Autodesk Inventor part; units mm, degrees
ref_plane "YZ Plane" through (0, 0, 0) normal (1, 0, 0) x (0, 1, 0)
ref_plane "XZ Plane" through (0, 0, 0) normal (0, 1, 0) x (-1, 0, 0)
ref_plane "XY Plane" through (0, 0, 0) normal (0, 0, 1) x (1, 0, 0)
sketch "Main Sketch" plane through (0, 0, 0) normal (0, 1, 0) x (-1, 0, 0)
  line L0 (-57.375, -12.0472) -> (-57.375, 12.0472)
  line L1 (-57.375, 12.0472) -> (47.625, -10) construction
  line L2 (47.625, 10) -> (-57.375, -12.0472) construction
  circle A0 centre (47.625, 0) radius 7
  line L3 (-40.875, 17.5) -> (-57.375, 17.5)
  line L4 (-57.375, 17.5) -> (-57.375, -17.5)
  line L5 (-57.375, -17.5) -> (-40.875, -17.5)
  line L6 (-40.875, 17.5) -> (-57.375, -17.5) construction
  line L7 (-57.375, 17.5) -> (-40.875, -17.5) construction
  line L8 (33.2636, -10) -> (-40.875, -10)
  line L9 (-40.875, -17.5) -> (-40.875, -10)
  line L10 (-40.875, 10) -> (-40.875, 17.5)
  line L11 (-40.875, 10) -> (33.2636, 10)
  arc A1 (33.2636, -10) -> (33.2636, 10) centre (47.625, 0) ccw
  point P0 (0, 0)
  point P1 (-49.125, 0)
  dimension "d3" = 14
  dimension "d13" = 16.5
  dimension "d14" = 35
  dimension "d15" = 0
  dimension "d18" = 20
  dimension "d101" = 35
extrude "Main Extrusion" add sketch "Main Sketch" along normal blind 4
sketch "Screw Holes Sketch" plane through (0, 4, 0) normal (0, 1, 0) x (1, 0, 0)
  circle A0 centre (46.125, -8.75) radius 2
  line L0 (57.375, 17.5) -> (40.875, 17.5)
  line L1 (40.875, -17.5) -> (57.375, -17.5)
  line L2 (35.2664, 0) -> (65.7891, 0)
  line L3 (51.375, -27.0398) -> (51.375, 30.2346) construction
  line L4 (57.375, -17.5) -> (57.375, 17.5)
  line L5 (40.875, -10) -> (40.875, -17.5)
  circle A1 centre (46.125, 8.75) radius 2
  line L6 (51.375, 27.0398) -> (51.375, -30.2346) construction
  point P0 (0, 0)
  dimension "d21" = 4
  dimension "d22" = 35
  dimension "d23" = 6
  dimension "d24" = 5.25
  dimension "d25" = 5.25
  dimension "d26" = 10.5
  dimension "d27" = 8.75
  dimension "d28" = 17.5
extrude "Screw Holes Cut" cut sketch "Screw Holes Sketch" against normal through all
fillet "Smoooooooooooooooooth" radius 6 2 edges at (40.875, 2, -17.5) (40.875, 2, 17.5)
sketch "Side Axel Hole Sketch" plane through (-47.625, 0, 10) normal (0, 0, 1) x (1, 0, 0)
  line L0 (88.5, 4) -> (88.5, 0)
  line L1 (0, 0) -> (0, 4)
  line L2 (44.25, -12.0383) -> (44.25, 22.7681) construction
  line L3 (14.3614, 0) -> (88.5, 0)
  line L4 (14.3614, 4) -> (88.5, 4)
  circle A0 centre (44.25, 4) radius 1.5
  point P0 (47.625, 0)
  dimension "d32" = 88.5
  dimension "d33" = 44.25
  dimension "d34" = 44.25
  dimension "d35" = 4
  dimension "d41" = 3
extrude "Side Axel Hole Cut" cut sketch "Side Axel Hole Sketch" against normal blind 20
sketch "Side Hole Extension Sketch" plane through (-47.625, 0, 10) normal (0, 0, 1) x (1, 0, 0)
  arc A0 (42.75, 4) -> (45.75, 4) centre (44.25, 4) ccw
  circle A1 centre (44.25, 4) radius 3
  circle A2 centre (44.25, 4) radius 1.5
  point P0 (47.625, 0)
  dimension "d44" = 6
extrude "Side Hole Extrusion" add sketch "Side Hole Extension Sketch" against normal blind 20
sketch "Body Holes Sketch" plane through (0, 4, 0) normal (0, 1, 0) x (1, 0, 0)
  line L0 (-37.625, 8) -> (-8.375, 8)
  line L1 (-8.375, 8) -> (-8.375, 4)
  line L2 (-8.375, 4) -> (-37.625, 4)
  line L3 (-37.625, 4) -> (-37.625, 8)
  line L4 (-6.375, -10) -> (-6.375, 10)
  circle A0 centre (-47.625, 0) radius 7
  line L5 (-47.625, 7) -> (-47.625, -13.5384) construction
  line L6 (-6.375, 10) -> (-0.375, 10)
  line L7 (-47.625, 1) -> (-47.625, -19.5384) construction
  line L8 (-37.625, 2) -> (-8.375, 2)
  line L9 (-8.375, 2) -> (-8.375, -2)
  line L10 (-8.375, -2) -> (-37.625, -2)
  line L11 (-37.625, -2) -> (-37.625, 2)
  line L12 (-47.625, -5) -> (-47.625, -25.5384) construction
  line L13 (-37.625, -4) -> (-8.375, -4)
  line L14 (-8.375, -4) -> (-8.375, -8)
  line L15 (-8.375, -8) -> (-37.625, -8)
  line L16 (-37.625, -8) -> (-37.625, -4)
  line L17 (1.625, 8) -> (39.625, 8)
  line L18 (39.625, 8) -> (39.625, 4)
  line L19 (39.625, 4) -> (1.625, 4)
  line L20 (1.625, 4) -> (1.625, 8)
  line L21 (-0.375, 10) -> (-0.375, -10)
  line L22 (40.875, 10) -> (-0.375, 10)
  line L23 (1.625, -2) -> (1.625, 2)
  line L24 (39.625, -2) -> (1.625, -2)
  line L25 (39.625, 2) -> (39.625, -2)
  line L26 (1.625, 2) -> (39.625, 2)
  line L27 (1.625, -8) -> (1.625, -4)
  line L28 (39.625, -8) -> (1.625, -8)
  line L29 (39.625, -4) -> (39.625, -8)
  line L30 (1.625, -4) -> (39.625, -4)
  point P0 (0, 0)
  point P1 (-47.625, 10)
  dimension "d86" = 10
  dimension "d77" = 4
  dimension "d78" = 2
  dimension "d79" = 10
  dimension "d80" = 2
  dimension "d83" = 6
  dimension "d88" = 2
  dimension "d89" = 2
  dimension "d90" = 4
  dimension "d91" = 38
  dimension "d94" = 6
extrude "Swiss-ified" cut sketch "Body Holes Sketch" against normal through all contours L0 L1 L2 L3 | L8 L9 L10 L11 | L13 L14 L15 L16 | L17 L18 L19 L20 | L23 L26 L25 L24 | L27 L30 L29 L28
sketch "Center Plate Attachment Sketch" plane through (0, 4, 0) normal (0, 1, 0) x (1, 0, 0)
  arc A0 (-33.2636, 10) -> (-33.2636, -10) centre (-47.625, 0) ccw construction
  line L0 (-47.625, 23.7347) -> (-47.625, -30.1469) construction
  circle A1 centre (-47.625, 13) radius 2
  circle A2 centre (-47.625, -13) radius 2
  circle A3 centre (-60.625, 0) radius 2
  point P0 (0, 0)
  dimension "d108" = 4
  dimension "d109" = 4
  dimension "d110" = 4
  dimension "d111" = 13
  dimension "d112" = 13
  dimension "d113" = 13
extrude "Center Plate Attachment Cut" cut sketch "Center Plate Attachment Sketch" against normal through all
properties part number "Side V3"
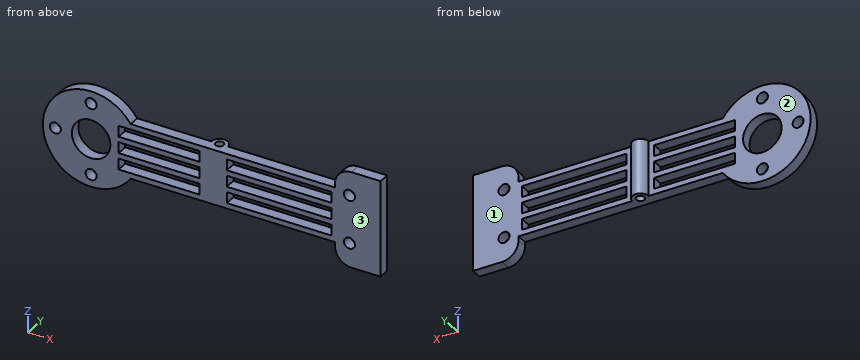
Work out the finished part from the listing and answer in its coordinate system (mm). Face numbers are marked on the shaded views. A direction names the side the tool comes from. Coordinates: 2 decimals unless noted, no trailing zeros. Loops run counter-clockwise (first coordinate to the right, second up) from the corner with the lowest first, then second, coordinate; pieces in that order, holes last. Notation, with made-up numbers: M 79,73 L 94,73 A9 ccw 94,84 Z; hole C 75.25,-37 d6. An arc over 180 degrees is marked long. Answer in a Markdown table with one row per item. Add a question column.
1. A tool of negligible diameter and unlimited length cuts with its end or side. For the marked faces 1, 2 and 3, from which of +Z, -Z, +X, -X, +Y, -Y can it reach the whole face along a straight path? Write none if from no direction.
2. Find section B-B, the plane x = 28. Write down the section's boundary in (y, z), then the cut area to 3 significant figures.
3. Find section C-C, the plane z = -13. Write down the section's boundary in (x, y) (3 decimals).
4. Flat-ended cylindrical pins translate along their axes: P1, Ø3, axis at x = -26.5, y = 1.5, coming from the +Z side; P2, Ø10.5, axis at x = -32.5, z = -1.5, coming from the +Y side; P3, Ø1.2, axis at y = 2.5, z = 6.5, coming from the -X side. Find the tip coordinate at first contact, or state that the pin passes through.
5. Consider L1, parallel to Z at x = 20, y = 1.5; L2, parallel to X at y = 1.2, z = 13 (3 decimals); L3, parallel to X at y = 4.5, z = 4. Determine where each line is inside the solid, lowest interval first.
6. Find section A-A, the plane z = 0. Write down the section's boundary in (x, y) (3 decimals), then the cut area to 3 significant figures.
Reported:
| question | item | result |
|---|---|---|
| 1 | face 1 | +Z, -Z, +X, +Y |
| 1 | face 2 | +Z, -Z, -X, +Y |
| 1 | face 3 | +Z, -Z, +X, -X, -Y |
| 2 | outline | M 0,-10 L 4,-10 L 4,-8 L 0,-8 Z; M 0,-4 L 4,-4 L 4,-2 L 0,-2 Z; M 0,2 L 4,2 L 4,4 L 0,4 Z; M 0,8 L 4,8 L 4,10 L 0,10 Z |
| 2 | area | 32.0 mm^2 |
| 3 | outline | M -59.34,0 L -49.625,0 L -49.625,4 L -59.34,4 Z; M -45.625,0 L -35.91,0 L -35.91,4 L -45.625,4 Z; M 41.066,0 L 57.375,0 L 57.375,4 L 41.066,4 Z |
| 4 | P1 | stops at z = 10 |
| 4 | P2 | stops at y = 4 |
| 4 | P3 | stops at x = -64.1 |
| 5 | L1 | z = -10 to -8, -4 to -2, 2 to 4, 8 to 10 |
| 5 | L2 | x = -59.34 to -49.625, -45.625 to -35.91, 41.066 to 57.375 |
| 5 | L3 | x = -6.33 to -4.79, -1.96 to -0.42 |
| 6 | outline | M -65.125,0 L -62.625,0 L -62.625,4 L -65.125,4 Z; M -58.625,0 L -54.625,0 L -54.625,4 L -58.625,4 Z; M -40.625,0 L -37.625,0 L -37.625,4 L -40.625,4 Z; M -8.375,0 L 1.625,0 L 1.625,4 L -0.375,4 A3 ccw -6.375,4 L -8.375,4 Z; M 39.625,0 L 57.375,0 L 57.375,4 L 39.625,4 Z; hole C -3.375,4 d3 |
| 6 | area | 156 mm^2 |
